Here's the drawing with two shaded views (mm, measured from the low corner). I have some questions. A direction names the side the tool comes from. Coordinates: 2 decimals unless noted, no trailing zeros. Write each loop counter-clockwise with the first axis right and the second up, starting at its lowest first coordinate (ties: lowest second). Pieces come first, ordered by that corner, then holes. Notation, with made-up numbers: (51.5, -37.5) - (87.5, -37.5) arc R17 cw to (87.5, -19.5) - close; hole circle Ø5 at (64, 40). An arc over 180 degrees is marked (long way). Answer in a Markdown table with one row per item. Add a question column.
Item 1: Imagine slicing it at C-C (x = 19.5). Please give me the cut outline in (y, z).
Item 2: Imagine slicing it at A-A (y = 30.65). Please give me the cut outline in (x, z), plus the area to 3 significant figures.
Item 3: Imagine slicing it at B-B (x = 55.3). Please give me the cut outline in (y, z) (1 decimal), plus the area to 3 significant figures.
Item 4: If I drill on probe 1 along Y at (x, z) = (31.75, 7); probe 2 along Z at (x, y) = (7.5, 13); probe 3 along Y at (x, z) = (17, 17.25) (1 decimal), over which ranges is the centre line in solid material (lowest first)? Write a range as from..to.
Item 5: Imagine slicing it at D-D (y = 44.5). Please give me the cut outline in (x, z).
Item 6: We'd pull the mould along Y, two halves only. Please class the marked faces 1, 2 and 3: +Y half, -Y half, draft (parallel to the pull), parting line (faces both ways), or undercut.
Item 7: Which directions (+Z, -Z, +X, -X, +Y, -Y) give clear straight access to the entire face, cutting with the end or side of a thin tool? Please do the marked faces 4, 5 and 6.
Item 8: I'm going to push flat-ended pins straight in: pin 1 (3 mm diameter, centred on x = 10.5, z = 14.5, fed in from -Y); pin 2 (6 mm diameter, centred on x = 18.32, y = 9.3, fed in from -Z); pin 3 (10 mm diameter, centred on x = 36, z = 4.5, fed in from -Y); pin 4 (3.5 mm diameter, centred on y = 38.15, z = 7, fed in from +X). Where does each tip first touch, or does it pass through?
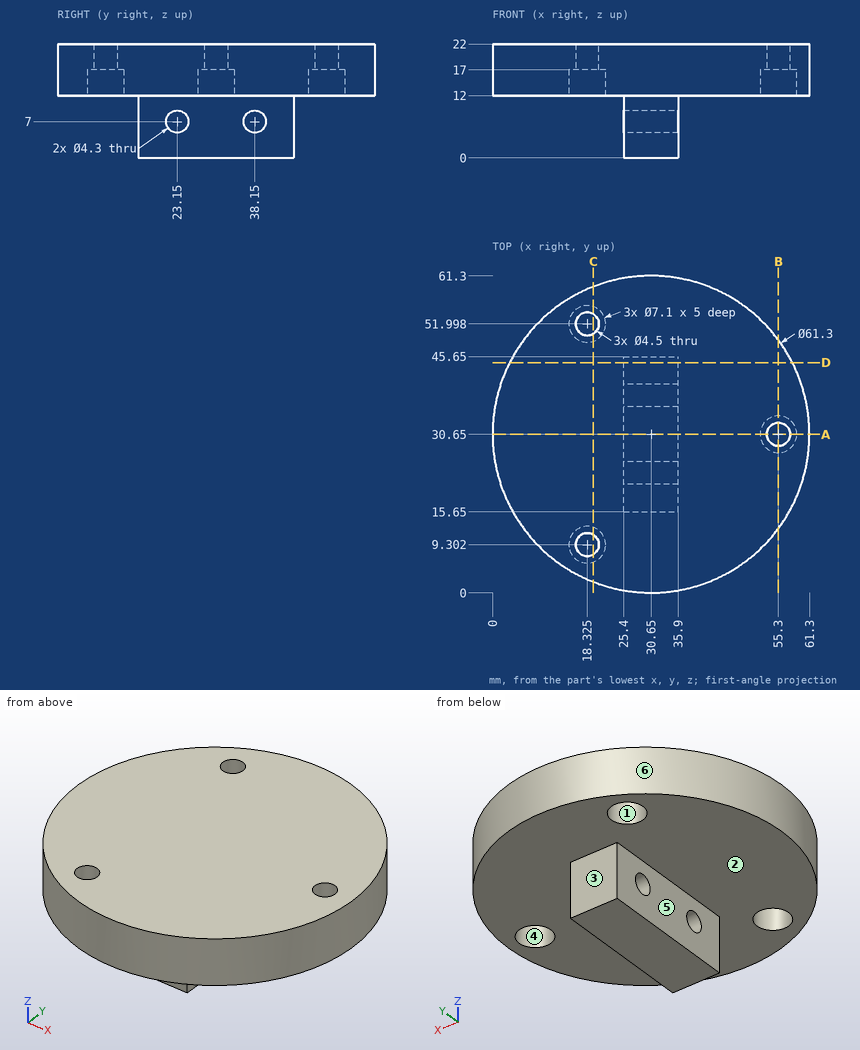
Here are the results:
| question | item | result |
|---|---|---|
| 1 | outline | (2.1, 12) - (5.95, 12) - (5.95, 17) - (7.38, 17) - (7.38, 22) - (2.1, 22) - close; (11.22, 17) - (12.65, 17) - (12.65, 12) - (48.65, 12) - (48.65, 17) - (50.08, 17) - (50.08, 22) - (11.22, 22) - close; (53.92, 17) - (55.35, 17) - (55.35, 12) - (59.2, 12) - (59.2, 22) - (53.92, 22) - close |
| 2 | outline | (0, 12) - (25.4, 12) - (25.4, 0) - (35.9, 0) - (35.9, 12) - (51.75, 12) - (51.75, 17) - (53.05, 17) - (53.05, 22) - (0, 22) - close; (57.55, 17) - (58.85, 17) - (58.85, 12) - (61.3, 12) - (61.3, 22) - (57.55, 22) - close |
| 2 | area | 681 mm2 |
| 3 | outline | (12.4, 12) - (27.1, 12) - (27.1, 17) - (28.4, 17) - (28.4, 22) - (12.4, 22) - close; (32.9, 17) - (34.2, 17) - (34.2, 12) - (48.9, 12) - (48.9, 22) - (32.9, 22) - close |
| 3 | area | 306 mm2 |
| 4 | probe 1 | y = 15.65..21, 25.3..36, 40.3..45.65 |
| 4 | probe 2 | z = 12..22 |
| 4 | probe 3 | y = 3.2..7.5, 11.1..50.2, 53.8..58.1 |
| 5 | outline | (3.31, 12) - (25.4, 12) - (25.4, 0) - (35.9, 0) - (35.9, 12) - (57.99, 12) - (57.99, 22) - (3.31, 22) - close |
| 6 | face 1 | undercut |
| 6 | face 2 | draft |
| 6 | face 3 | +Y half |
| 7 | face 4 | -Z |
| 7 | face 5 | -Z, -X, +Y, -Y |
| 7 | face 6 | +Z, -Z |
| 8 | pin 1 | stops at y = 6.33 |
| 8 | pin 2 | stops at z = 17 |
| 8 | pin 3 | stops at y = 15.65 |
| 8 | pin 4 | passes through |
